The figure shows three views and two pictorial views of one solid part (mm, origin at its lowest corner). Answer the questions. A direction names the side the tool comes from. Give positions to 0.01 mm unless a question says otherwise; leave off trailing zeros. Loops run counter-clockwise (first coordinate to the right, second up) from the corner with the lowest first, then second, coordinate; pieces in that order, holes last. Notation, with made-up numbers: (50.25, 46.25) - (108.25, 46.25) arc R16 cw to (108.25, 51.25) - close; hole circle Ø1 at (87, 66). An arc over 180 degrees is marked (long way). Write each question's results on one line, items separated by ' | '.
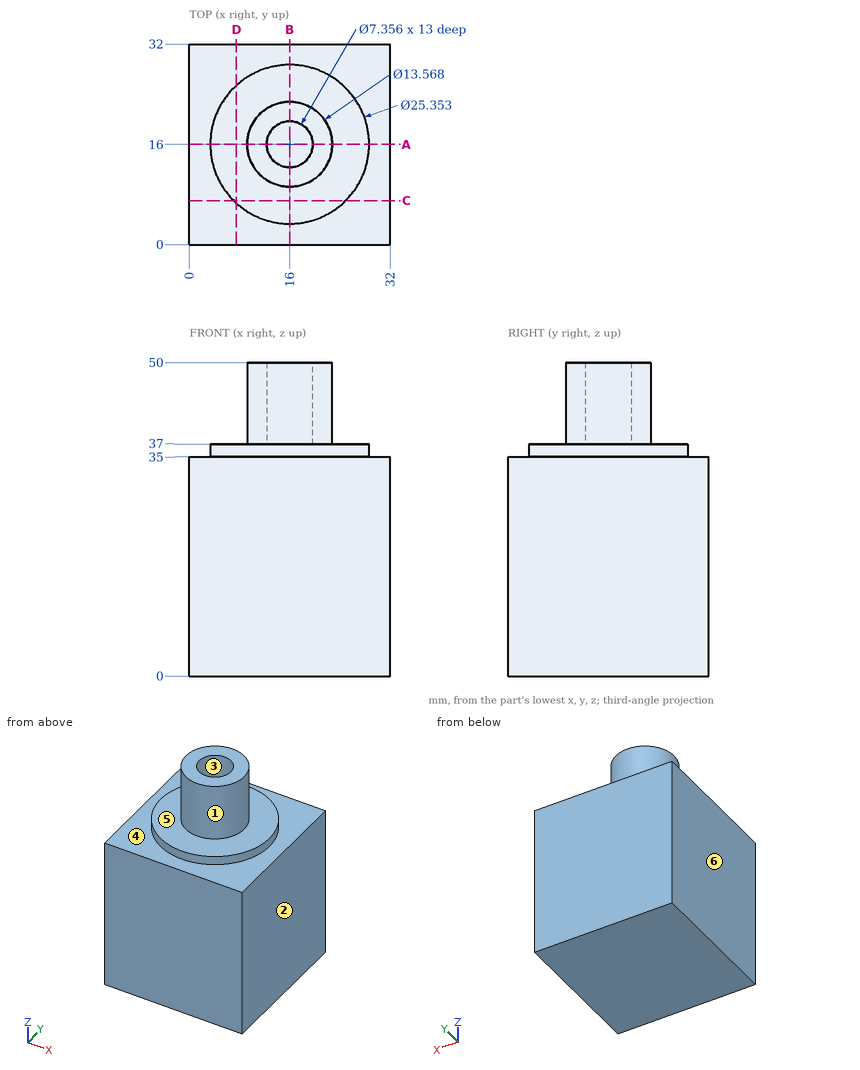
Item 1: A cutting plane is placed at D-D, the plane x = 7.5. Determine the outline of the cut face in (y, z) (1 decimal), plus the area to 3 significant figures.
Values found:
outline: (0, 0) - (32, 0) - (32, 35) - (25.4, 35) - (25.4, 37) - (6.6, 37) - (6.6, 35) - (0, 35) - close | area: 1,160 mm²
Item 2: For the marked faces 5 and 6, determine the directions among +Z, -Z, +X, -X, +Y, -Y from which every point of the face is accessible in a straight line to the end or side of a thin tool.
Values found:
face 5: +Z | face 6: +Z, -Z, -X, +Y, -Y
Item 3: A cutting plane is placed at C-C, the plane y = 7. Determine the outline of the cut face in (x, z), plus the area to 3 significant figures.
Values found:
outline: (0, 0) - (32, 0) - (32, 35) - (24.93, 35) - (24.93, 37) - (7.07, 37) - (7.07, 35) - (0, 35) - close | area: 1,160 mm²
Item 4: For a pull along X with two mould halves and no side action, classify the marked faces 1, 2, 3 and 4 as released by +X, released by -X, zero draft, split by the parting line, or undercut.
Values found:
face 1: split by the parting line | face 2: released by +X | face 3: undercut | face 4: zero draft
Item 5: A cutting plane is placed at A-A, the plane y = 16. Determine the outline of the cut face in (x, z).
Values found:
outline: (0, 0) - (32, 0) - (32, 35) - (28.68, 35) - (28.68, 37) - (22.78, 37) - (22.78, 50) - (19.68, 50) - (19.68, 37) - (12.32, 37) - (12.32, 50) - (9.22, 50) - (9.22, 37) - (3.32, 37) - (3.32, 35) - (0, 35) - close
Item 6: Find the intervals of material crossed by line 1 along Y through (x, z) = (16, 44.75); line 2 along Z through (x, y) = (13, 30.5), in increasing order. Write a range as [from, to].
Values found:
line 1: y = [9.22, 12.32], [19.68, 22.78] | line 2: z = [0, 35]
Item 7: A flat-ended cylindrical pin translates along its axis: P1, Ø2, axis at x = 17.5, y = 14.5, coming from the +Z side. Find the tip coordinate at first contact, or state that the pin passes through.
Values found:
P1: stops at z = 37
